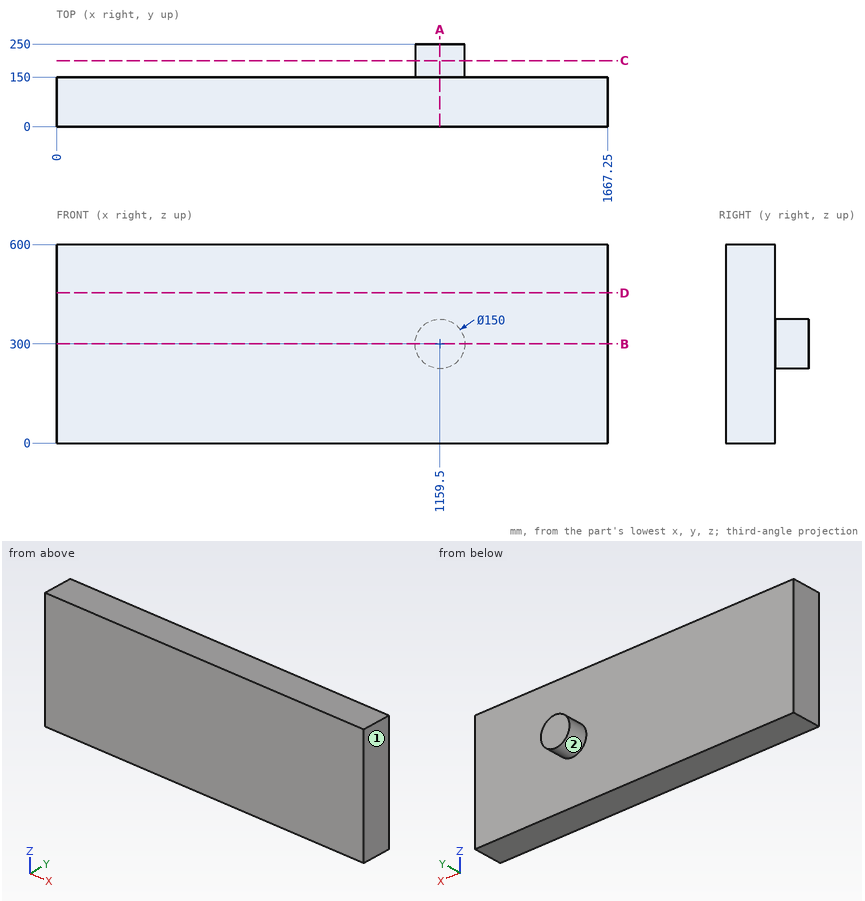
Verification items for this drawing (mm, ordinates from the low corner). A direction names the side the tool comes from. Coordinates: 2 decimals unless noted, no trailing zeros. Order: outer loops, then holes, each group sorted by start corner. A loop starts at its lowest first (then second) coordinate and runs counter-clockwise, first axis right, second up. Notation, with made-up numbers: (-5, -30) - (43, -30) arc R9 cw to (43, -19) - close; hole circle Ø3 at (89.5, -13). An arc over 180 degrees is marked (long way). Answer as a JSON object with one key per item and string values. Group by question number.
Item 1: Sectioned sample at D-D, the plane z = 454. Record the cut outline in (x, y), and give its area (3 significant figures).
Item 2: Sectioned sample at A-A, the plane x = 1159.5. Record the cut outline in (y, z), and give its area (3 significant figures).
Item 3: Depth check by flat-ended pin: pin 1 Ø4 at (x, y) = (1201, 157.5) entering from +Z; pin 2 Ø5 at (y, z) = (178.5, 322.5) entering from -X. Enter the tip coordinate at first touch or a pass-through.
Item 4: Sectioned sample at C-C, the plane y = 199.5. Record the cut outline in (x, z).
Item 5: Tool access check on the marked faces 1 and 2. Record the directions out of +Z, -Z, +X, -X, +Y, -Y that give a thin tool (end or side, any length) a straight path to the whole face; none if there is none.
Item 6: Sectioned sample at B-B, the plane z = 300. Record the cut outline in (x, y).
Item 7: Scan lines: probe 1 along Y at (x, z) = (247.5, 399.5); probe 2 along X at (y, z) = (161, 239). Record each from-to range of solid material in increasing order.
Resolved:
{
 "1": {"outline": "(0, 0) - (1667.25, 0) - (1667.25, 150) - (0, 150) - close", "area": "250,000 mm^2"},
 "2": {"outline": "(0, 0) - (150, 0) - (150, 225) - (250, 225) - (250, 375) - (150, 375) - (150, 600) - (0, 600) - close", "area": "105,000 mm^2"},
 "3": {"pin 1": "z = 363.76", "pin 2": "x = 1087.22"},
 "4": {"outline": "circle Ø150 at (1159.5, 300)"},
 "5": {"face 1": "+Z, -Z, +X, +Y, -Y", "face 2": "+Y"},
 "6": {"outline": "(0, 0) - (1667.25, 0) - (1667.25, 150) - (1234.5, 150) - (1234.5, 250) - (1084.5, 250) - (1084.5, 150) - (0, 150) - close"},
 "7": {"probe 1": "0 to 150", "probe 2": "1115.87 to 1203.13"}
}
